For this review, take the finished solid that the model builds, in its own axes (mm). A direction names the side the tool comes from. Round coordinates to 2 decimals unless told otherwise and drop trailing zeros. Write each loop counter-clockwise with the first axis right and the second up, starting at its lowest first coordinate (ties: lowest second). Pieces come first, ordered by that corner, then holes. Notation, with made-up numbers: M 61.5,-31.75 L 71.5,-31.75 A15 cw 71.5,-6.75 Z; hole C 19,28 d9. An arc over 180 degrees is marked long. Write each question's results on one line, items separated by ' | '. Start each with the question number.
```python
from build123d import *

# Parameters (mm, degrees)
SKETCH2_W           = 96
SKETCH2_H           = 30
SKETCH2_R           = 1.5
BOSS_EXTRUDE2_DEPTH = 10
BOSS_EXTRUDE4_DEPTH = 100
BOSS_EXTRUDE5_DEPTH = 26
LPATTERN1_COUNT     = 2
LPATTERN1_PITCH     = 50


with BuildPart() as part:
    # Sketch2 → Boss-Extrude2 (new body)
    with BuildSketch(Plane(origin=(0, 0, 0), x_dir=(1, 0, 0), z_dir=(0, 1, 0))):
        with Locations((0, 119.85)):
            Rectangle(SKETCH2_W, SKETCH2_H)
        with Locations((-30, 127)):
            Circle(SKETCH2_R, mode=Mode.SUBTRACT)
        with Locations((30, 127)):
            Circle(SKETCH2_R, mode=Mode.SUBTRACT)
    extrude(amount=BOSS_EXTRUDE2_DEPTH)

    # Sketch4 → Boss-Extrude4 (add)
    with BuildSketch(Plane(origin=(0, 0, 0), x_dir=(1, 0, 0), z_dir=(0, 1, 0))):
        with BuildLine():
            Line((-22.15, 134.85), (22.15, 134.85))
            Line((22.15, 134.85), (22.15, 127))
            ThreePointArc((22.15, 127), (24.449211768, 121.449211768), (30, 119.15))
            Line((30, 119.15), (48, 119.15))
            Line((48, 119.15), (48, 104.85))
            Line((48, 104.85), (-48, 104.85))
            Line((-48, 104.85), (-48, 119.15))
            Line((-48, 119.15), (-30, 119.15))
            ThreePointArc((-30, 119.15), (-24.449211768, 121.449211768), (-22.15, 127))
            Line((-22.15, 127), (-22.15, 134.85))
        make_face()
    extrude(amount=BOSS_EXTRUDE4_DEPTH)

    # Sketch6 → Boss-Extrude5 (add)
    with BuildSketch(Plane(origin=(0, 100, 0), x_dir=(1, 0, 0), z_dir=(0, 1, 0))):
        with BuildLine():
            Line((22.15, 134.85), (22.15, 104.85))
            Line((22.15, 104.85), (-22.15, 104.85))
            Line((-22.15, 104.85), (-22.15, 134.85))
            ThreePointArc((-22.15, 134.85), (0, 159.85), (22.15, 134.85))
        make_face()
    boss_extrude5 = extrude(amount=-BOSS_EXTRUDE5_DEPTH)

    # LPattern1: Boss-Extrude5 ×2
    with Locations(*[(0, -i * LPATTERN1_PITCH, 0) for i in range(1, LPATTERN1_COUNT)]):
        add(boss_extrude5)


solid = part.part
```
Item 1: We need section C-C on x = 0. State the section outline as (y, z) points, then the cut area to 3 significant figures.
Item 2: We need section A-A on z = -143. State the section outline as (x, y) points, then the cut area to 3 significant figures.
Item 3: Mouldability with a two-part tool opening along Y and no side actions: class faces 1 (the flat face through (-22.15, 54, -131)), 2 (the flat face through (-35, 10, -127)), 3 (the flat face through (0, 50, -145)) as pulls with the +Y half, pulls with the -Y half, needs draft (parallel to the pull), parting line crosses it, or undercut.
Item 4: Insertion check: P1, Ø14.5, axis at x = 38.5, y = 46.5, coming from the -Z side; P2, Ø7.5, axis at x = -3, z = -145.5, coming from the -Y side; P3, Ø5, axis at y = 36.5, z = -143.5, coming from the +X side; P4, Ø1.8, axis at x = 30, z = -127, coming from the +Y side. Each pin has a flat end and moves straight along its axis. Give the tip position at first contact, or say it passes through.
Item 5: For faces 4 (the flat face through (-1, 9, -134.85)), 5 (the flat face through (39, 54, -119.15)), 6 (the flat face through (0, 74, -145)), 7 (the flat face through (-39, 54, -119.15)), list the 3-axis set-ups (+Z, -Z, +X, -X, +Y, -Y) from which the entire face can be reached by the end or side of a thin tool; tool diameter is ignored.
Item 6: We need section D-D on z = -121. State the section outline as (x, y) points.
Item 7: We need section B-B on y = 68.5. State the section outline as (x, z) points, then the cut area to 3 significant figures.
Item 8: For probe 1 along X at (y, z) = (2.5, -127); probe 2 along Z at (x, y) = (30, 4.25); probe 3 along Y at (x, z) = (-19, -142), list the stretches that pass through material, from the lowest coordinate up.
Numbers:
1) outline: M 0,-134.85 L 24,-134.85 L 24,-159.85 L 50,-159.85 L 50,-134.85 L 74,-134.85 L 74,-159.85 L 100,-159.85 L 100,-104.85 L 0,-104.85 Z | area: 4,300 mm^2
2) outline: M -21.63,24 L 21.63,24 L 21.63,50 L -21.63,50 Z; M -21.63,74 L 21.63,74 L 21.63,100 L -21.63,100 Z | area: 2,250 mm^2
3) face 1: needs draft | face 2: pulls with the +Y half | face 3: undercut
4) P1: stops at z = -119.15 | P2: stops at y = 24 | P3: stops at x = 22.04 | P4: passes through
5) face 4: -Z, +X, -X, -Y | face 5: -Z, +X, +Y | face 6: -Z, +X, -X | face 7: -Z, -X, +Y
6) outline: M -48,0 L 48,0 L 48,10 L 24.94,10 L 24.94,100 L -24.94,100 L -24.94,10 L -48,10 Z
7) outline: M -48,-119.15 L -30,-119.15 A7.85 cw -22.15,-127 L -22.15,-134.85 L 22.15,-134.85 L 22.15,-127 A7.85 cw 30,-119.15 L 48,-119.15 L 48,-104.85 L -48,-104.85 Z | area: 2,090 mm^2
8) probe 1: x = -48 to -31.5, -28.5 to 28.5, 31.5 to 48 | probe 2: z = -134.85 to -128.5, -125.5 to -104.85 | probe 3: y = 24 to 50, 74 to 100
